Verification items for the finished model (mm, model axes). Face numbers are marked on the shaded views. A direction names the side the tool comes from. Give positions to 0.01 mm unless a question says otherwise; leave off trailing zeros. Loops run counter-clockwise (first coordinate to the right, second up) from the corner with the lowest first, then second, coordinate; pieces in that order, holes last. Notation, with made-up numbers: (47, -39) - (75, -39) arc R10 cw to (75, -27) - close; hole circle Ø11 at (65.5, 10). An arc over 180 degrees is marked (long way). Put each result on its own line as item: value. Start each with the question number.
```python
from build123d import *

# Parameters (mm, degrees)
F1_DEPTH = 25.4
F2_W     = 24
F2_H     = 10
F3_DEPTH = 20


with BuildPart() as f1:
    # F0 (on Top) → F1 (new body)
    with BuildSketch(Plane.XY):
        Polygon((90, 0), (0, 0), (0, -40), (52, -78), (90, -78), align=None)
    extrude(amount=F1_DEPTH)

    # F2 (on face) → F3 (join)
    with BuildSketch(Plane.XZ.offset(78)):
        with Locations((34.221601, 12.58618)):
            Rectangle(F2_W, F2_H)
    extrude(amount=-F3_DEPTH)


solid = f1.part
```
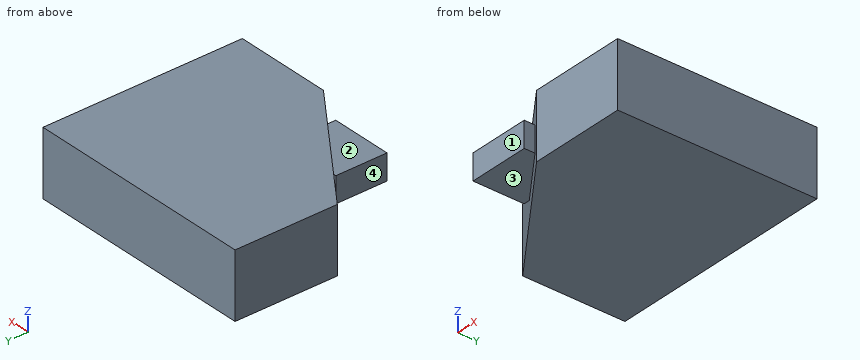
1) Section check A-A, the plane x = 32.5. Enter the section's corners in (y, z).
2) Section check C-C, the plane y = -60. Enter the section's corners in (x, z).
3) Scan lines: line 1 along X through (y, z) = (-69, 14); line 2 along X through (y, z) = (-43, 16); line 3 along Y through (x, z) = (21, 9.5). Record each from-to range of solid material in increasing order. Write a range as from..to.
4) Section check B-B, the plane z = 19. Enter the section's corners in (x, y).
5) Depth check by flat-ended pin: P1, Ø2.5, axis at x = 23, z = 13.5, coming from the +Y side; P2, Ø3, axis at y = -66, z = 11, coming from the -X side; P3, Ø10, axis at y = -48, z = 14.5, coming from the -X side. Enter the tip coordinate at first touch or a pass-through.
6) Section check D-D, the plane z = 12.25. Enter the section's corners in (x, y).
7) Set-up check for the marked faces 1, 2, 3 and 4: record each of +Z, -Z, +X, -X, +Y, -Y from which the full face is reachable in a straight line by a thin tool's end or side.
Results are:
1. outline: (-78, 7.59) - (-63.75, 7.59) - (-63.75, 0) - (0, 0) - (0, 25.4) - (-63.75, 25.4) - (-63.75, 17.59) - (-78, 17.59) - close
2. outline: (22.22, 7.59) - (27.37, 7.59) - (27.37, 0) - (90, 0) - (90, 25.4) - (27.37, 25.4) - (27.37, 17.59) - (22.22, 17.59) - close
3. line 1: x = 22.22..90
3. line 2: x = 4.11..90
3. line 3: y = -55.35..0
4. outline: (0, -40) - (52, -78) - (90, -78) - (90, 0) - (0, 0) - close
5. P1: stops at y = 0
5. P2: stops at x = 22.22
5. P3: stops at x = 4.11
6. outline: (0, -40) - (24.63, -58) - (22.22, -58) - (22.22, -78) - (46.22, -78) - (46.22, -73.78) - (52, -78) - (90, -78) - (90, 0) - (0, 0) - close
7. face 1: +Z, -Z, +X, -X, -Y
7. face 2: +Z, -X, -Y
7. face 3: -Z, -X, -Y
7. face 4: +Z, -Z, -X, -Y
